Check sheet for the modelled part. Datum: model origin and axes. Units: mm. A direction names the side the tool comes from. Round coordinates to 2 decimals unless told otherwise and drop trailing zeros. Loops run counter-clockwise (first coordinate to the right, second up) from the corner with the lowest first, then second, coordinate; pieces in that order, holes last. Notation, with made-up numbers: (-2.5, 61.5) - (30.5, 61.5) arc R35 cw to (30.5, 94.5) - close; hole circle Ø7 at (-39, 43). An arc over 180 degrees is marked (long way). Put each result on its own line as item: value.
```python
from build123d import *

# Parameters (mm, degrees)
BOX004_W                  = 11.5
BOX004_H                  = 49
BOX004_DEPTH              = 8
BOX003_W                  = 22
BOX003_H                  = 49
BOX003_DEPTH              = 3.3
FILLET001_R               = 1
BOX005_W                  = 15
BOX005_H                  = 49
BOX005_DEPTH              = 3
BOX001_W                  = 30.5
BOX001_H                  = 12
BOX001_DEPTH              = 2.25
CYLINDER_R                = 2.7
CYLINDER_DEPTH            = 10
BOX002_W                  = 15
BOX002_H                  = 12
BOX002_DEPTH              = 2.25
FILLET_R                  = 2
FUSION001_PLACEMENT_ANGLE = 180
CYLINDER001_R             = 2.7
CYLINDER001_DEPTH         = 10
BOX_W                     = 120
BOX_H                     = 12
BOX_DEPTH                 = 80
FILLET002_R               = 0.5
ARRAY_Y_COUNT             = 4
ARRAY_Y_PITCH             = 12.2
BOX006_W                  = 40
BOX006_H                  = 49
BOX006_DEPTH              = 15
FILLET003_R               = 1


with BuildPart() as box004:
    # Box004 → Box004 (new body)
    with BuildSketch(Plane(origin=(-38, -0.2, 84.5), x_dir=(1, 0, 0), z_dir=(0, 0, 1))):
        with Locations((5.75, 24.5)):
            Rectangle(BOX004_W, BOX004_H)
    extrude(amount=BOX004_DEPTH)


with BuildPart() as fillet001:
    # Box003 → Box003 (new body)
    with BuildSketch(Plane(origin=(-43, -0.2, 84.5), x_dir=(1, 0, 0), z_dir=(0, 0, 1))):
        with Locations((11, 24.5)):
            Rectangle(BOX003_W, BOX003_H)
    extrude(amount=BOX003_DEPTH)

    # Fillet001
    fillet001_edges = [fillet001.edges().sort_by_distance(p)[0] for p in [
        (-43, -0.2, 86.15),
        (-43, 48.8, 86.15),
        (-21, -0.2, 86.15),
        (-21, 48.8, 86.15),
    ]]
    fillet(fillet001_edges, radius=FILLET001_R)


with BuildPart() as fusion002005:
    # Box005 → Box005 (new body)
    with BuildSketch(Plane(origin=(-39.5, -0.2, 82), x_dir=(1, 0, 0), z_dir=(0, 0, 1))):
        with Locations((7.5, 24.5)):
            Rectangle(BOX005_W, BOX005_H)
    extrude(amount=BOX005_DEPTH)

    # Fusion002005: union Box004, Fillet001
    add(box004.part)
    add(fillet001.part)


with BuildPart() as obj1:
    # Box001 → Box001 (new body)
    with BuildSketch(Plane.XY):
        with Locations((15.25, 6)):
            Rectangle(BOX001_W, BOX001_H)
    extrude(amount=BOX001_DEPTH)


with BuildPart() as cylinder:
    # Cylinder → Cylinder (new body)
    with BuildSketch(Plane(origin=(7.5, 6, 4.5), x_dir=(1, 0, 0), z_dir=(0, 0, 1))):
        Circle(CYLINDER_R)
    extrude(amount=CYLINDER_DEPTH)


with BuildPart() as fillet_body:
    # Box002 → Box002 (new body)
    with BuildSketch(Plane.XY.offset(2.25)):
        with Locations((7.5, 6)):
            Rectangle(BOX002_W, BOX002_H)
    extrude(amount=BOX002_DEPTH)

    # Fillet
    fillet_edges = [fillet_body.edges().sort_by_distance(p)[0] for p in [
        (0, 6, 4.5),
        (15, 6, 4.5),
    ]]
    fillet(fillet_edges, radius=FILLET_R)


with BuildPart() as fusion001:
    # Fusion001 base: copy of Fillet body
    add(fillet_body.part)

    # Fusion001: union obj1, Cylinder
    add(obj1.part)
    add(cylinder.part)


with BuildPart() as fusion001_1:
    # Fusion001 placement: moved
    add(fusion001.part.moved(Location((-24.5, 12, 80))).rotate(Axis((-24.5, 12, 80), (0, 0, 1)), FUSION001_PLACEMENT_ANGLE))


with BuildPart() as cylinder001:
    # Cylinder001 → Cylinder001 (new body)
    with BuildSketch(Plane(origin=(7.5, 6, 4.5), x_dir=(1, 0, 0), z_dir=(0, 0, 1))):
        Circle(CYLINDER001_R)
    extrude(amount=CYLINDER001_DEPTH)


with BuildPart() as fillet002:
    # Box → Box (new body)
    with BuildSketch(Plane(origin=(-84.5, 0, -80), x_dir=(1, 0, 0), z_dir=(0, 0, 1))):
        with Locations((60, 6)):
            Rectangle(BOX_W, BOX_H)
    extrude(amount=BOX_DEPTH)

    # Fillet002
    fillet002_edges = [fillet002.edges().sort_by_distance(p)[0] for p in [
        (-84.5, 0, -40),
        (-84.5, 6, 0),
        (-84.5, 12, -40),
        (-84.5, 6, -80),
        (35.5, 0, -40),
        (35.5, 6, 0),
        (35.5, 12, -40),
        (35.5, 6, -80),
        (-24.5, 0, -80),
        (-24.5, 0, 0),
        (-24.5, 12, -80),
        (-24.5, 12, 0),
    ]]
    fillet(fillet002_edges, radius=FILLET002_R)


with BuildPart() as fusion002006:
    # Fusion base: copy of Fillet body
    add(fillet_body.part)

    # Fusion: union obj1, Cylinder, Fillet002
    add(obj1.part)
    add(cylinder.part)
    add(fillet002.part)


with BuildPart() as fusion002006_1:
    # Fusion placement: moved
    add(fusion002006.part.moved(Location((24.5, 0, 80))))

    # Fusion002: union Fusion001, Cylinder001
    add(fusion001_1.part)
    add(cylinder001.part)

    # Array Y: Fusion002006 ×4


with BuildPart() as fusion002006_2:
    add(fusion002006_1.part)
    with Locations(*[(0, i * ARRAY_Y_PITCH, 0) for i in range(1, ARRAY_Y_COUNT)]):
        add(fusion002006_1.part)

    # Fusion002006: union Fusion002005
    add(fusion002005.part)


with BuildPart() as cut:
    # Box006 → Box006 (new body)
    with BuildSketch(Plane(origin=(-58, -0.2, 80.5), x_dir=(1, 0, 0), z_dir=(0, 0, 1))):
        with Locations((20, 24.5)):
            Rectangle(BOX006_W, BOX006_H)
    extrude(amount=BOX006_DEPTH)

    # Fillet003
    fillet003_edges = [cut.edges().sort_by_distance(p)[0] for p in [
        (-58, -0.2, 88),
        (-58, 48.8, 88),
        (-18, -0.2, 88),
        (-18, 48.8, 88),
    ]]
    fillet(fillet003_edges, radius=FILLET003_R)

    # Cut: cut Fusion002006
    add(fusion002006_2.part, mode=Mode.SUBTRACT)


solid = cut.part
```
Item 1: Go/stop test with flat-tipped pins: pin 1 (4.5 mm diameter, centred on x = -32, y = 30.5, fed in from -Z); pin 2 (9.5 mm diameter, centred on x = -50, y = 7, fed in from -Z). Record where each tip stops, or that it passes through.
Filled sheet:
pin 1: z = 94.5
pin 2: z = 82.25
Item 2: Thickness scan on line 1 (Y direction, x = -32, z = 94.1); line 2 (Y direction, x = -37, z = 81.5); line 3 (X direction, y = 16.5, z = 85). Record the ranges inside material, lowest first. Write a range as from..to.
Filled sheet:
line 1: -0.2..3.3, 8.7..15.5, 20.9..27.7, 33.1..39.9, 45.3..48.8
line 2: -0.2..0, 12..12.2, 24.2..24.4, 36.4..36.6, 48.6..48.8
line 3: -58..-43, -21..-18
Item 3: Section check C-C on y = 22. Enter the section's corners in (x, z).
Filled sheet:
outline: (-58, 80.5) - (-55, 80.5) - (-55, 82.25) - (-39.5, 82.25) - (-39.5, 84.5) - (-43, 84.5) - (-43, 87.8) - (-38, 87.8) - (-38, 92.5) - (-26.5, 92.5) - (-26.5, 87.8) - (-21, 87.8) - (-21, 84.5) - (-24.5, 84.5) - (-24.5, 80.5) - (-18, 80.5) - (-18, 95.5) - (-58, 95.5) - close
Item 4: Release check for a two-part mould opening along X. For faces 1 (the cylindrical face through (-57.715, 48.499, 88.105)), 2 (the flat face through (-55, 6, 81)), 3 (the flat face through (-23, 23, 80.5)) record: +X half, -X half, draft (parallel to the pull), parting line (faces both ways), or undercut.
Filled sheet:
face 1: -X half
face 2: undercut
face 3: draft
Item 5: Tool access check on faces 4 (the flat face through (-58, 24, 88)), 5 (the flat face through (-21, 24, 86)), 6 (the flat face through (-32, 6, 94.5)). Record the directions out of +Z, -Z, +X, -X, +Y, -Y that give a thin tool (end or side, any length) a straight path to the whole face; none if there is none.
Filled sheet:
face 4: +Z, -Z, -X, +Y, -Y
face 5: none
face 6: -Z
Item 6: Section check A-A on z = 87. Enter the section's corners in (x, y).
Filled sheet:
outline: (-58, 0.8) arc R1 ccw to (-57, -0.2) - (-42, -0.2) arc R1 cw to (-43, 0.8) - (-43, 47.8) arc R1 cw to (-42, 48.8) - (-57, 48.8) arc R1 ccw to (-58, 47.8) - close; (-22, -0.2) - (-19, -0.2) arc R1 ccw to (-18, 0.8) - (-18, 47.8) arc R1 ccw to (-19, 48.8) - (-22, 48.8) arc R1 cw to (-21, 47.8) - (-21, 0.8) arc R1 cw to start
Item 7: Section check B-B on x = -46. Enter the section's corners in (y, z).
Filled sheet:
outline: (-0.2, 80.5) - (0, 80.5) - (0, 82.25) - (12, 82.25) - (12, 80.5) - (12.2, 80.5) - (12.2, 82.25) - (24.2, 82.25) - (24.2, 80.5) - (24.4, 80.5) - (24.4, 82.25) - (36.4, 82.25) - (36.4, 80.5) - (36.6, 80.5) - (36.6, 82.25) - (48.6, 82.25) - (48.6, 80.5) - (48.8, 80.5) - (48.8, 95.5) - (-0.2, 95.5) - close
Item 8: Section check D-D on x = -32. Count the separate pieces of the cut face and the enclosed holes in it, then the cut area to 3 significant figures.
Filled sheet:
separate pieces: 6
enclosed holes: 0
area: 105 mm²
